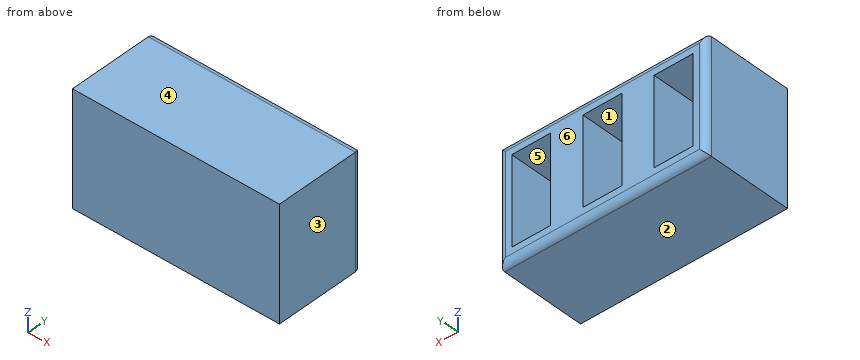
```python
from build123d import *

# Parameters (mm, degrees)
SKETCH1_W           = 32
SKETCH1_H           = 17.5
BOSS_EXTRUDE1_DEPTH = 14
SKETCH2_W           = 6
SKETCH2_H           = 13.5
CUT_EXTRUDE1_DEPTH  = 13.6
LPATTERN1_COUNT     = 3
LPATTERN1_PITCH     = 11
FILLET1_R           = 1


with BuildPart() as part:
    # Sketch1 → Boss-Extrude1 (new body)
    with BuildSketch(Plane(origin=(0, 0, 0), x_dir=(1, 0, 0), z_dir=(0, 1, 0))):
        with Locations((16, 8.75)):
            Rectangle(SKETCH1_W, SKETCH1_H)
    extrude(amount=BOSS_EXTRUDE1_DEPTH)

    # Sketch2 → Cut-Extrude1 (cut)
    with BuildSketch(Plane(origin=(0, 14, 0), x_dir=(1, 0, 0), z_dir=(0, 1, 0))):
        with Locations((5, 8.75)):
            Rectangle(SKETCH2_W, SKETCH2_H)
    cut_extrude1 = extrude(amount=-CUT_EXTRUDE1_DEPTH, mode=Mode.SUBTRACT)

    # LPattern1: Cut-Extrude1 ×3
    with Locations(*[(i * LPATTERN1_PITCH, 0, 0) for i in range(1, LPATTERN1_COUNT)]):
        add(cut_extrude1, mode=Mode.SUBTRACT)

    # Fillet1
    fillet1_edges = [part.edges().sort_by_distance(p)[0] for p in [
        (32, 14, -8.75),
        (16, 14, -17.5),
        (0, 14, -8.75),
        (16, 14, 0),
    ]]
    fillet(fillet1_edges, radius=FILLET1_R)


solid = part.part
```
Build history of the part. All positions in model axes, mm. Face numbers are marked on the shaded views. A direction names the side the tool comes from. Give positions to 0.01 mm unless a question says otherwise; leave off trailing zeros. Loops run counter-clockwise (first coordinate to the right, second up) from the corner with the lowest first, then second, coordinate; pieces in that order, holes last. Notation, with made-up numbers: (89, -14.75) - (142, -14.75) arc R27 ccw to (142, 13.25) - close; hole circle Ø3 at (-2.5, 68.5). An arc over 180 degrees is marked (long way). Use a Markdown table: item, result.
(1) Wall check: line 1 along X through (y, z) = (2.75, -12); line 2 along Z through (x, y) = (18.5, 1); line 3 along Y through (x, z) = (18.5, -10.25). Give the ranges that are in metal, low to high.
Taken from the geometry:
| item | result |
|---|---|
| line 1 | 0 to 2, 8 to 13, 19 to 24, 30 to 32 |
| line 2 | -17.5 to -15.5, -2 to 0 |
| line 3 | 0 to 0.4 |
(2) Pull direction Z, two halves, no side cores. Call the marked faces 1, 2, 3 and 4: +Z half, -Z half, draft (parallel to the pull), parting line (faces both ways), or undercut.
Taken from the geometry:
| item | result |
|---|---|
| face 1 | undercut |
| face 2 | -Z half |
| face 3 | draft |
| face 4 | +Z half |
(3) Band-saw the part on A-A (y = 9.5). Give the cut face in (x, z), and give its area (3 significant figures).
Taken from the geometry:
| item | result |
|---|---|
| outline | (0, -17.5) - (32, -17.5) - (32, 0) - (0, 0) - close; hole (2, -15.5) - (8, -15.5) - (8, -2) - (2, -2) - close; hole (13, -15.5) - (19, -15.5) - (19, -2) - (13, -2) - close; hole (24, -15.5) - (30, -15.5) - (30, -2) - (24, -2) - close |
| area | 317 mm2 |
(4) Band-saw the part on B-B (z = -9.5). Give the cut face in (x, y), and give its area (3 significant figures).
Taken from the geometry:
| item | result |
|---|---|
| outline | (0, 0) - (32, 0) - (32, 13) arc R1 ccw to (31, 14) - (30, 14) - (30, 0.4) - (24, 0.4) - (24, 14) - (19, 14) - (19, 0.4) - (13, 0.4) - (13, 14) - (8, 14) - (8, 0.4) - (2, 0.4) - (2, 14) - (1, 14) arc R1 ccw to (0, 13) - close |
| area | 203 mm2 |
(5) Which spindle directions (+Z, -Z, +X, -X, +Y, -Y) get a long thin tool onto all of the face, cutting with end or side? Do the marked faces 5 and 6. Say none if no direction does.
Taken from the geometry:
| item | result |
|---|---|
| face 5 | +Y |
| face 6 | +Z, -Z, +X, -X, +Y |
(6) Band-saw the part on C-C (x = 27.5). Give the cut face in (y, z), and give its area (3 significant figures).
Taken from the geometry:
| item | result |
|---|---|
| outline | (0, -17.5) - (13, -17.5) arc R1 ccw to (14, -16.5) - (14, -15.5) - (0.4, -15.5) - (0.4, -2) - (14, -2) - (14, -1) arc R1 ccw to (13, 0) - (0, 0) - close |
| area | 61.0 mm2 |
